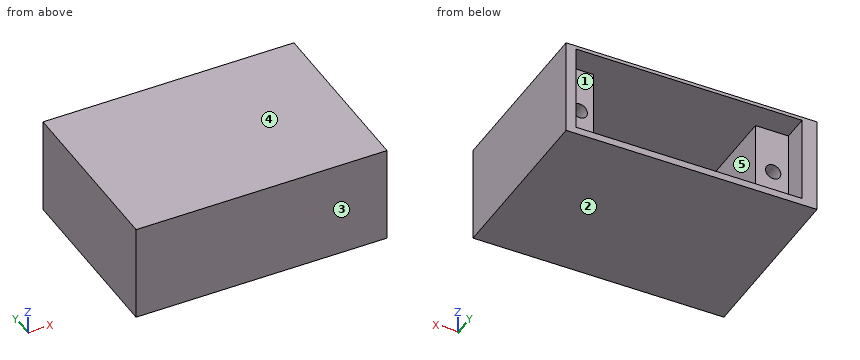
```python
from build123d import *

# Parameters (mm, degrees)
CYLINDER004_R     = 1.1
CYLINDER004_DEPTH = 10
CYLINDER005_R     = 1.1
CYLINDER005_DEPTH = 10
SKETCH007_W       = 23.3
SKETCH007_H       = 12.5
PAD007_DEPTH      = 19.5
SKETCH005_W       = 32.5
SKETCH005_H       = 12.5
PAD006_DEPTH      = 4.5
SKETCH006_W       = 36.061928
SKETCH006_H       = 25.639376
PAD005_DEPTH      = 14


with BuildPart() as cylinder004:
    # Cylinder004 → Cylinder004 (new body)
    with BuildSketch(Plane(origin=(30, 22, 6), x_dir=(1, 0, 0), z_dir=(0, -1, 0))):
        Circle(CYLINDER004_R)
    extrude(amount=CYLINDER004_DEPTH)


with BuildPart() as obj1:
    # Cylinder005 → Cylinder005 (new body)
    with BuildSketch(Plane(origin=(2.2, 22, 6), x_dir=(1, 0, 0), z_dir=(0, -1, 0))):
        Circle(CYLINDER005_R)
    extrude(amount=CYLINDER005_DEPTH)

    # Fusion003: union Cylinder004
    add(cylinder004.part)


with BuildPart() as cortecuerpo001:
    # Sketch007 → Pad007 (new body)
    with BuildSketch(Plane.XZ):
        with Locations((16.4, 6.25)):
            Rectangle(SKETCH007_W, SKETCH007_H)
    extrude(amount=PAD007_DEPTH)


with BuildPart() as cortecuerpo001_1:
    # Body009 placement: moved
    add(cortecuerpo001.part.moved(Location((0, 19, 0))))


with BuildPart() as cortetornillos001:
    # Sketch005 → Pad006 (new body)
    with BuildSketch(Plane.XZ):
        with Locations((16.25, 6.25)):
            Rectangle(SKETCH005_W, SKETCH005_H)
    extrude(amount=PAD006_DEPTH)


with BuildPart() as cortetornillos001_1:
    # Body008 placement: moved
    add(cortetornillos001.part.moved(Location((0, 23, 0))))


with BuildPart() as obj2:
    # Sketch006 → Pad005 (new body)
    with BuildSketch(Plane.XY):
        with Locations((15.881367, 9.413649)):
            Rectangle(SKETCH006_W, SKETCH006_H)
    extrude(amount=PAD005_DEPTH)


with BuildPart() as obj2_1:
    # Body007 placement: moved
    add(obj2.part.moved(Location((0, 0, -1))))

    # Cut003: cut CorteTornillos001
    add(cortetornillos001_1.part, mode=Mode.SUBTRACT)

    # Cut004: cut CorteCuerpo001
    add(cortecuerpo001_1.part, mode=Mode.SUBTRACT)

    # Cut005: cut obj1
    add(obj1.part, mode=Mode.SUBTRACT)


solid = obj2_1.part
```
Can you work these out from the model? Positions are in its coordinate system, mm. Face numbers are marked on the shaded views. A direction names the side the tool comes from. Give positions to 0.01 mm unless a question says otherwise; leave off trailing zeros. Loops run counter-clockwise (first coordinate to the right, second up) from the corner with the lowest first, then second, coordinate; pieces in that order, holes last. Notation, with made-up numbers: M -9,22.5 L 41,22.5 A14 cw 41,47.5 Z; hole C -33.5,-13 d7. An arc over 180 degrees is marked long. Use one line per item in the form item = value. Start each with the question number.
(1) I want a section at B-B, the plane y = 13.25. Write out the boundary of the cut face in (x, z).
(2) On a 3-axis mill with a long thin cutter (end or side, diameter ignored), from which of +Z, -Z, +X, -X, +Y, -Y can I reach the whole of each face in a straight line? I mean the marked faces 1 and 2. Say none if no direction works.
(3) Thinking about a two-plate mould opening in Z: for the marked faces 3, 4 and 5, which applies, released by +Z, released by -Z, zero draft, split by the parting line, or undercut?
(4) I want a section at A-A, the plane y = 20.25. Write out the boundary of the cut face in (x, z), and give its area (3 significant figures).
(5) I'm going to push flat-ended pins straight in: P1, Ø6, axis at x = 19, z = 8.5, coming from the +Y side; P2, Ø1.1, axis at x = 30, z = 6.5, coming from the +Y side; P3, Ø2.5, axis at x = 3.5, z = 3.5, coming from the +Y side. Where does each tip first touch, or does it pass through?
(6) Please list where these lines run through material, in increasing order: line 1 (X direction, y = 14.5, z = 6); line 2 (Z direction, x = 21, y = 20.25); line 3 (X direction, y = 8, z = 1.75).
(7) I want a section at D-D, the plane x = 2.2. Write out the boundary of the cut face in (y, z), and give its area (3 significant figures).
(8) I want a section at C-C, the plane z = 6. Write out the boundary of the cut face in (x, y).
Worked out:
q1.outline = M -2.15,-1 L 33.91,-1 L 33.91,13 L -2.15,13 Z; hole C 2.2,6 d2.2; hole M 4.75,0 L 28.05,0 L 28.05,12.5 L 4.75,12.5 Z; hole C 30,6 d2.2
q2.face_1 = +Y
q2.face_2 = -Z, +X, -X, +Y, -Y
q3.face_3 = zero draft
q3.face_4 = released by +Z
q3.face_5 = undercut
q4.outline = M -2.15,-1 L 33.91,-1 L 33.91,13 L -2.15,13 Z; hole M 0,0 L 32.5,0 L 32.5,12.5 L 0,12.5 Z
q4.area = 98.6 mm²
q5.P1 = -0.5
q5.P2 = 12
q5.P3 = 18.5
q6.line_1 = -2.15 to 1.1, 3.3 to 4.75, 28.05 to 28.9, 31.1 to 33.91
q6.line_2 = -1 to 0, 12.5 to 13
q6.line_3 = -2.15 to 4.75, 28.05 to 33.91
q7.outline = M -3.41,-1 L 22.23,-1 L 22.23,0 L 18.5,0 L 18.5,4.9 L 12,4.9 L 12,7.1 L 18.5,7.1 L 18.5,12.5 L 22.23,12.5 L 22.23,13 L -3.41,13 Z
q7.area = 298 mm²
q8.outline = M -2.15,-3.41 L 33.91,-3.41 L 33.91,22.23 L 32.5,22.23 L 32.5,18.5 L 31.1,18.5 L 31.1,12 L 28.9,12 L 28.9,18.5 L 28.05,18.5 L 28.05,-0.5 L 4.75,-0.5 L 4.75,18.5 L 3.3,18.5 L 3.3,12 L 1.1,12 L 1.1,18.5 L 0,18.5 L 0,22.23 L -2.15,22.23 Z
